Could you check a few things on this model? Use its own coordinates, in mm. Face numbers are marked on the shaded views. A direction names the side the tool comes from. Coordinates: 2 decimals unless noted, no trailing zeros. Order: outer loops, then holes, each group sorted by start corner. A loop starts at its lowest first (then second) coordinate and runs counter-clockwise, first axis right, second up. Notation, with made-up numbers: (14.25, 45.25) - (70.25, 45.25) arc R22 cw to (70.25, 74.25) - close; hole circle Ø9 at (-31.75, -8.5). An arc over 180 degrees is marked (long way). Answer as CSV lines item,"result". Start each with the question number.
1. I want a section at D-D, the plane x = -15. List the corners of the cut face in (y, z) for me (3 decimals), and give its area (3 significant figures).
2. I need wall thicknesses on probe 1 along Y at (x, z) = (10, -12.55) (3 decimals); probe 2 along X at (y, z) = (-1.75, -4); probe 3 along Z at (x, y) = (21, 0) (1 decimal). Which ranges of each line are inside material? Lowest first, please.
3. For pin 1 (4 mm diameter, centred on x = 0, y = 4, fed in from +Z) (3 decimals); pin 2 (1.5 mm diameter, centred on y = -4, z = -4, fed in from +X); pin 3 (1.2 mm diameter, centred on y = 2.5, z = 12.5, fed in from +X); pin 4 (1.8 mm diameter, centred on y = 0, z = 6, fed in from +X), each with a flat end and sliding along its axis, tell me the tip position at first contact or that it passes through.
4. I want a section at A-A, the plane x = -10. List the corners of the cut face in (y, z) for me (3 decimals).
5. Thinking about a two-plate mould opening in Z: for the marked faces 3, 4, 5 and 6, which applies, released by +Z, released by -Z, zero draft, split by the parting line, or undercut?
6. I want a section at B-B, the plane z = -9. List the corners of the cut face in (x, y) for me (3 decimals).
7. I want a section at C-C, the plane z = 6. Count the separate pieces of the cut face and the enclosed holes in it, and give its area (3 significant figures).
8. For the marked faces 1 and 2, which set-ups out of +Z, -Z, +X, -X, +Y, -Y let a thin tool reach every point of the face, with its end or its side?
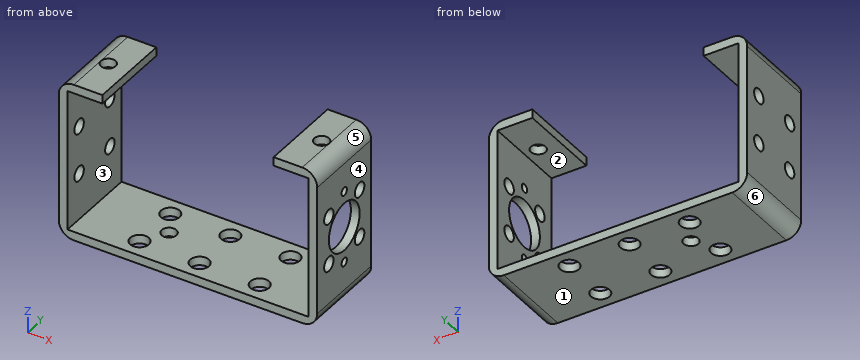
Solid Edge part; units mm, degrees
sketch "Sketch1" plane through (0, 0, 0) normal (0, -1, 0) x (1, 0, 0)
  line L0 (-21.5, 13.225) -> (21.5, 13.225)
  line L1 (21.5, 13.225) -> (21.5, -13.225)
  line L2 (21.5, -13.225) -> (-21.5, -13.225)
  line L3 (-21.5, -13.225) -> (-21.5, 13.225)
  line L4 (-20.05, 11.775) -> (20.05, 11.775)
  line L5 (20.05, 11.775) -> (20.05, -11.775)
  line L6 (20.05, -11.775) -> (-20.05, -11.775)
  line L7 (-20.05, -11.775) -> (-20.05, 11.775)
  dimension "D1" = 21.5
  dimension "D2" = 21.5
extrude "Protrusion1" add sketch "Sketch1" along normal mid plane 14.05
sketch "Sketch2" plane through (0, -7.025, 0) normal (0, -1, 0) x (1, 0, 0)
  line L0 (-14.25, 13.225) -> (14.25, 13.225)
  line L1 (14.25, 13.225) -> (14.25, 11.775)
  line L2 (14.25, 11.775) -> (-14.25, 11.775)
  line L3 (-14.25, 11.775) -> (-14.25, 13.225)
  dimension "D1" = 14.25
extrude "Cutout1" cut sketch "Sketch2" against normal up to next
hole "Hole_1" at (-17.75, 0, 13.225) direction (0, 0, -1) diameter 2.459 end up to next
hole "Hole1" at (17.75, 0, 13.225) direction (0, 0, -1) diameter 2.459 end up to next
hole "Hole_3" at (10, -4, -13.225) direction (0, 0, 1) diameter 3.1 end up to next
hole "Hole2" at (10, 4, -13.225) direction (0, 0, 1) diameter 3.1 end up to next
hole "Hole3" at (0, 4, -13.225) direction (0, 0, 1) diameter 3.1 end up to next
hole "Hole4" at (0, -4, -13.225) direction (0, 0, 1) diameter 3.1 end up to next
hole "Hole5" at (-10, -4, -13.225) direction (0, 0, 1) diameter 3.1 end up to next
hole "Hole6" at (-10, 4, -13.225) direction (0, 0, 1) diameter 3.1 end up to next
hole "Hole_9" at (-21.5, 4, 4) direction (1, 0, 0) diameter 2.459 end through all
hole "Hole7" at (-21.5, -4, 4) direction (1, 0, 0) diameter 2.459 end through all
hole "Hole8" at (-21.5, -4, -4) direction (1, 0, 0) diameter 2.459 end through all
hole "Hole9" at (-21.5, 4, -4) direction (1, 0, 0) diameter 2.459 end through all
fillet "Round_1" radius 2.5 4 edges at (-21.5, 0, 13.225) (-21.5, 0, -13.225) (21.5, 0, -13.225) (21.5, 0, 13.225)
hole "Hole_13" at (21.5, 0, 0) direction (-1, 0, 0) diameter 8 end up to next
hole "Hole_14" at (21.5, 0, 6) direction (-1, 0, 0) diameter 1.383 end up to next
hole "Hole10" at (21.5, 0, -6) direction (-1, 0, 0) diameter 1.383 end up to next
hole "Hole_16" at (-7.65, 0, -13.225) direction (0, 0, 1) diameter 2.459 end up to next
Solved:
1,outline,"(-7.025, -13.225) - (7.025, -13.225) - (7.025, -11.775) - (-7.025, -11.775) - close; (-7.025, 11.775) - (7.025, 11.775) - (7.025, 13.225) - (-7.025, 13.225) - close"
1,area,"40.7 mm2"
2,probe 1,"y = -7.025 to -5.55, -2.45 to 2.45, 5.55 to 7.025"
2,probe 2,"x = -21.5 to -20.05, 20.05 to 21.5"
2,probe 3,"z = -12.2 to -6.7, -5.3 to -4, 4 to 5.3, 6.7 to 12.2"
3,pin 1,"stops at z = -11.775"
3,pin 2,"passes through"
3,pin 3,"stops at x = 21.21"
3,pin 4,"stops at x = 21.5"
4,outline,"(-7.025, -13.225) - (-5.55, -13.225) - (-5.55, -11.775) - (-7.025, -11.775) - close; (-2.45, -13.225) - (2.45, -13.225) - (2.45, -11.775) - (-2.45, -11.775) - close; (5.55, -13.225) - (7.025, -13.225) - (7.025, -11.775) - (5.55, -11.775) - close"
5,face 3,"undercut"
5,face 4,"zero draft"
5,face 5,"released by +Z"
5,face 6,"released by -Z"
6,outline,"(-21.5, -7.025) - (-20.05, -7.025) - (-20.05, 7.025) - (-21.5, 7.025) - close; (20.05, -7.025) - (21.5, -7.025) - (21.5, 7.025) - (20.05, 7.025) - close"
7,separate pieces,"3"
7,enclosed holes,"0"
7,area,"38.7 mm2"
8,face 1,"-Z, +X, -X, +Y, -Y"
8,face 2,"+Y, -Y"
